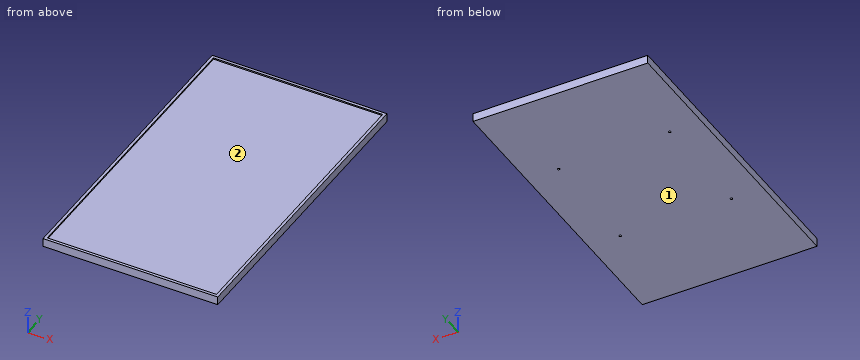
from build123d import *

# Parameters (mm, degrees)
SKETCH1_W           = 629.1
SKETCH1_H           = 1096.9
BOSS_EXTRUDE1_DEPTH = 30.5
SKETCH2_R           = 4
CUT_EXTRUDE1_DEPTH  = 21
SKETCH3_W           = 609.1
SKETCH3_H           = 1076.9
CUT_EXTRUDE2_DEPTH  = 5


with BuildPart() as part:
    # Sketch1 → Boss-Extrude1 (new body)
    with BuildSketch(Plane.XY):
        Rectangle(SKETCH1_W, SKETCH1_H)
    extrude(amount=BOSS_EXTRUDE1_DEPTH)

    # Sketch2 → Cut-Extrude1 (cut)
    with BuildSketch(Plane(origin=(0, 0, 0), x_dir=(-1, 0, 0), z_dir=(0, 0, -1))):
        with Locations((-200, 200)):
            Circle(SKETCH2_R)
        with Locations((200, 200)):
            Circle(SKETCH2_R)
        with Locations((200, -200)):
            Circle(SKETCH2_R)
        with Locations((-200, -200)):
            Circle(SKETCH2_R)
    extrude(amount=-CUT_EXTRUDE1_DEPTH, mode=Mode.SUBTRACT)

    # Sketch3 → Cut-Extrude2 (cut)
    with BuildSketch(Plane.XY.offset(30.5)):
        Rectangle(SKETCH3_W, SKETCH3_H)
    extrude(amount=-CUT_EXTRUDE2_DEPTH, mode=Mode.SUBTRACT)


solid = part.part
Read the model definition and answer for the solid it produces. Units are mm, in the model's axes. Face numbers are marked on the shaded views. Coordinates: 2 decimals unless noted, no trailing zeros. Write each loop counter-clockwise with the first axis right and the second up, starting at its lowest first coordinate (ties: lowest second). Pieces come first, ordered by that corner, then holes. Notation, with made-up numbers: (6, -23.75) - (33, -23.75) arc R15 cw to (33, -19.75) - close; hole circle Ø9 at (37.5, 35). An arc over 180 degrees is marked (long way). One line per question, with ' | ' between items.
Q1. Find section A-A, the plane y = -416.5. Write down the section's boundary in (x, z).
Result set:
outline: (-314.55, 0) - (314.55, 0) - (314.55, 30.5) - (304.55, 30.5) - (304.55, 25.5) - (-304.55, 25.5) - (-304.55, 30.5) - (-314.55, 30.5) - close
Q2. Determine the mould class of the marked faces 1 and 2 for opening direction Y: +Y half, -Y half, draft (parallel to the pull), parting line (faces both ways), or undercut.
Result set:
face 1: draft | face 2: undercut
Q3. Consider L1, parallel to Y at x = -200, z = 9.5; L2, parallel to X at y = 409, z = 27; L3, parallel to Y at x = -134, z = 28. Determine where each line is inside the solid, lowest interval first. Write a range as [from, to].
Result set:
L1: [-548.45, -204], [-196, 196], [204, 548.45] | L2: [-314.55, -304.55], [304.55, 314.55] | L3: [-548.45, -538.45], [538.45, 548.45]
Q4. Each of these flat-tipped pins is pushed along its axis until it touches: P1, Ø9, axis at x = -200, y = -200, coming from the -Z side; P2, Ø6.5, axis at x = -200, y = 200, coming from the +Z side; P3, Ø7, axis at x = 200, y = 200, coming from the -Z side. Where does it stop, or does it pass through?
Result set:
P1: z = 0 | P2: z = 25.5 | P3: z = 21
